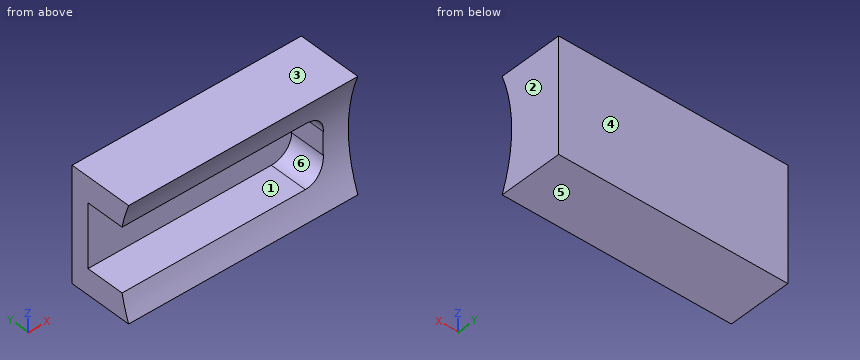
```python
from build123d import *

# Parameters (mm, degrees)
SKETCH1_W           = 18
SKETCH1_H           = 9
BOSS_EXTRUDE1_DEPTH = 5
CUT_EXTRUDE1_DEPTH  = 20.215878851
CUT_EXTRUDE3_DEPTH  = 3.6


with BuildPart() as part:
    # Sketch1 → Boss-Extrude1 (new body)
    with BuildSketch(Plane(origin=(0, 0, 0), x_dir=(1, 0, 0), z_dir=(0, 1, 0))):
        Rectangle(SKETCH1_W, SKETCH1_H)
    extrude(amount=BOSS_EXTRUDE1_DEPTH)

    # Sketch2 → Cut-Extrude1 (cut, through all)
    with BuildSketch(Plane.ZY.offset(9)):
        with BuildLine():
            Line((-4.5, 0), (4.5, 0))
            ThreePointArc((4.5, 0), (0, 0.83809621), (-4.5, 0))
        make_face()
    extrude(amount=-CUT_EXTRUDE1_DEPTH, mode=Mode.SUBTRACT)

    # Sketch3 → Cut-Extrude3 (cut)
    with BuildSketch(Plane(origin=(0, 0, 0), x_dir=(1, 0, 0), z_dir=(0, 1, 0))):
        with BuildLine():
            Line((-9, 2.5), (5.4, 2.5))
            ThreePointArc((5.4, 2.5), (6.53137085, 2.03137085), (7, 0.9))
            Line((7, 0.9), (7, -0.9))
            ThreePointArc((7, -0.9), (6.53137085, -2.03137085), (5.4, -2.5))
            Line((5.4, -2.5), (-9, -2.5))
            Line((-9, -2.5), (-9, 2.5))
        make_face()
    extrude(amount=CUT_EXTRUDE3_DEPTH, mode=Mode.SUBTRACT)


solid = part.part
```
Geometry: final body of the model. Coordinates: model frame, mm. Face numbers are marked on the shaded views. A direction names the side the tool comes from. Coordinates: 2 decimals unless noted, no trailing zeros. Order: outer loops, then holes, each group sorted by start corner. A loop starts at its lowest first (then second) coordinate and runs counter-clockwise, first axis right, second up. Notation, with made-up numbers: (33.25, 58) - (42.25, 58) arc R17 cw to (42.25, 74) - close; hole circle Ø7 at (-21, 44.25). An arc over 180 degrees is marked (long way). Return JSON: item names as keys, results as strings. Group by question number.
1. Pin query (flat end, axial travel): pin 1 (4 mm diameter, centred on x = 2.5, z = 1, fed in from -Y); pin 2 (0.5 mm diameter, centred on y = 1.5, z = 0, fed in from -X); pin 3 (1.5 mm diameter, centred on x = -1.5, z = -3.5, fed in from -Y). Return the tip coordinate at first contact, or that it passes through.
2. Cut plane B-B (x = -5.5). Output: boundary loops of the cut face in (y, z), plus the area to 3 significant figures.
3. Cut plane C-C (z = 1.5). Output: boundary loops of the cut face in (x, y), plus the area to 3 significant figures.
4. Cut plane D-D (x = 5.75). Output: boundary loops of the cut face in (y, z).
5. Cut plane A-A (y = 2.3). Output: boundary loops of the cut face in (x, z).
6. Material intervals for line 1 along Z through (x, y) = (-3.75, 1.15); line 2 along Y through (x, z) = (-1.25, -0.5); line 3 along Y through (x, z) = (6, -2.5), sorted ascending. Write a range as [from, to].
7. Pull-direction query (Z, two-part tool) for the marked faces 3, 4, 5 and 6; classes: pulls with the +Z half, pulls with the -Z half, needs draft (parallel to the pull), parting line crosses it, or undercut.
8. Set-up query: the marked faces 1 and 2. Return all of +Z, -Z, +X, -X, +Y, -Y with unobstructed straight access to the full face (end or side cutting, diameter ignored); none if empty.
Resolved:
{
 "1": {"pin 1": "stops at y = 0.47", "pin 2": "stops at x = 7", "pin 3": "stops at y = 0.09"},
 "2": {"outline": "(0, -4.5) - (5, -4.5) - (5, 4.5) - (0, 4.5) arc R12.5 cw to (0.59, 2.5) - (3.6, 2.5) - (3.6, -2.5) - (0.59, -2.5) arc R12.5 cw to start", "area": "25.7 mm²"},
 "3": {"outline": "(-9, 3.6) - (6.88, 3.6) - (6.88, 0.75) - (9, 0.75) - (9, 5) - (-9, 5) - close", "area": "31.2 mm²"},
 "4": {"outline": "(0, -4.5) - (5, -4.5) - (5, 4.5) - (0, 4.5) arc R12.5 cw to (0.59, 2.46) - (3.6, 2.46) - (3.6, -2.46) - (0.59, -2.46) arc R12.5 cw to start"},
 "5": {"outline": "(-9, -4.5) - (9, -4.5) - (9, 4.5) - (-9, 4.5) - (-9, 2.5) - (5.4, 2.5) arc R1.6 cw to (7, 0.9) - (7, -0.9) arc R1.6 cw to (5.4, -2.5) - (-9, -2.5) - close"},
 "6": {"line 1": "z = [-4.5, -2.5], [2.5, 4.5]", "line 2": "y = [3.6, 5]", "line 3": "y = [0.59, 5]"},
 "7": {"face 3": "pulls with the +Z half", "face 4": "needs draft", "face 5": "pulls with the -Z half", "face 6": "undercut"},
 "8": {"face 1": "-X, -Y", "face 2": "+Z, -Z, +X, +Y, -Y"}
}
